The listing builds one solid part. Answer for the finished solid, in the listing's coordinates (mm). A direction names the side the tool comes from. Coordinates: 2 decimals unless noted, no trailing zeros. Order: outer loops, then holes, each group sorted by start corner. A loop starts at its lowest first (then second) coordinate and runs counter-clockwise, first axis right, second up.
from build123d import *

# Parameters (mm, degrees)
EXTRUDE_1_DEPTH     = 16
FILLET_1_R          = 8
SKETCH_2_R          = 2.5
CUT_EXTRUDE_1_DEPTH = 16
SKETCH_3_R          = 2.5
CUT_EXTRUDE_2_DEPTH = 16
CHAMFER_1_SIZE      = 1
FILLET_2_R          = 1


with BuildPart() as part:
    # 草图1 → 凸台-拉伸1 (new body)
    with BuildSketch(Plane.XY):
        Polygon((0, 38), (0, 0), (-38, 0), (-38, -2), (2, -2), (2, 38), align=None)
    extrude(amount=EXTRUDE_1_DEPTH)

    # 圆角1
    fillet_1_edges = [part.edges().sort_by_distance(p)[0] for p in [
        (-38, -1, 0),
        (-38, -1, 16),
        (1, 38, 16),
        (1, 38, 0),
    ]]
    fillet(fillet_1_edges, radius=FILLET_1_R - 0.0001)  # a hair under: the kernel refuses the full size

    # 草图2 → 切除-拉伸1 (cut)
    with BuildSketch(Plane.ZY):
        with Locations(Location((8, 30, 0), (0, 0, 270))):
            Circle(SKETCH_2_R)
        with Locations(Location((8, 8, 0), (0, 0, 270))):
            Circle(SKETCH_2_R)
    extrude(amount=-CUT_EXTRUDE_1_DEPTH, mode=Mode.SUBTRACT)

    # 草图3 → 切除-拉伸2 (cut)
    with BuildSketch(Plane(origin=(0, 0, 0), x_dir=(1, 0, 0), z_dir=(0, 1, 0))):
        with Locations(Location((-30, -8, 0), (0, 0, 180))):
            Circle(SKETCH_3_R)
        with Locations(Location((-8, -8, 0), (0, 0, 180))):
            Circle(SKETCH_3_R)
    extrude(amount=-CUT_EXTRUDE_2_DEPTH, mode=Mode.SUBTRACT)

    # 倒角1
    chamfer_1_edges = [part.edges().sort_by_distance(p)[0] for p in [
        (0, 32.5, 8),
        (0, 10.5, 8),
        (-27.5, 0, 8),
        (-5.5, 0, 8),
    ]]
    chamfer(chamfer_1_edges, length=CHAMFER_1_SIZE)

    # 圆角2
    fillet_2_edges = [part.edges().sort_by_distance(p)[0] for p in [
        (2, -2, 8),
        (0, 0, 8),
    ]]
    fillet(fillet_2_edges, radius=FILLET_2_R)


solid = part.part
(1) Find section A-A on x = -8. Determine the outline of the cut face in (y, z).
(2) A tool of negligible diameter and unlimited length cuts with its end or side. For faces 1 (the cylindrical face through (1.715, -1.699, 8.112)), 2 (the flat face through (-19, 0, 8)), from which of +Z, -Z, +X, -X, +Y, -Y can it reach the whole face along a straight path? Write none if from no direction.
(3) Find section D-D on y = 13. Determine the outline of the cut face in (x, z).
(4) Find section C-C on z = 12.5. Determine the outline of the cut face in (x, y), then the cut area to 3 significant figures.
(5) Find section B-B on z = 7.5. Count the separate pieces of the cut face and the enclosed holes in it, then the cut area to 3 significant figures.
(6) The mould has two halves that part along X. Classify faces 3 (the cylindrical face through (0.986, 35.719, 13.594)), 4 (the cylindrical face through (-28, -1.5, 6.5)), 5 (the flat face through (2, 18, 8)), 6 (the cylindrical face through (-35.719, -1.014, 2.406)): pulls with the +X half, pulls with the -X half, needs draft (parallel to the pull), parting line crosses it, or undercut.
(7) Find the intervals of material crossed by probe 1 along Z at (x, y) = (-8, -1.75); probe 2 along Y at (x, z) = (-10.5, 5.25); probe 3 along X at (y, z) = (1.5, 2.75), in increasing order.
(8) Given pin 1 Ø6 at (y, z) = (8, 8) entering from -X; pin 2 Ø3 at (y, z) = (33.5, 5) entering from -X; pin 3 Ø4 at (x, z) = (-33, 4.5) entering from +Y, each flat-ended and moving along its own axis, determine where each tip first touches the part or whether it passes through.
Resolved:
1. outline: (-2, 0) - (0, 0) - (0, 4.5) - (-1, 5.5) - (-2, 5.5) - close; (-2, 10.5) - (-1, 10.5) - (0, 11.5) - (0, 16) - (-2, 16) - close
2. face 1: +Z, -Z, +X, -Y
2. face 2: +Z, -Z, -X, +Y
3. outline: (0, 0) - (2, 0) - (2, 16) - (0, 16) - close
4. outline: (-36.61, -2) - (1, -2) arc R1 ccw to (2, -1) - (2, 36.61) - (0, 36.61) - (0, 1) arc R1 cw to (-1, 0) - (-36.61, 0) - close
4. area: 150 mm2
5. separate pieces: 5
5. enclosed holes: 0
5. area: 113 mm2
6. face 3: needs draft
6. face 4: undercut
6. face 5: pulls with the +X half
6. face 6: pulls with the -X half
7. probe 1: z = 0 to 5.5, 10.5 to 16
7. probe 2: y = -2 to 0
7. probe 3: x = 0 to 2
8. pin 1: stops at x = 0.5
8. pin 2: stops at x = 0
8. pin 3: stops at y = 0
